The listing builds one solid part. Answer for the finished solid, in the listing's coordinates (mm). A direction names the side the tool comes from. Round coordinates to 2 decimals unless told otherwise and drop trailing zeros. Order: outer loops, then holes, each group sorted by start corner. A loop starts at its lowest first (then second) coordinate and runs counter-clockwise, first axis right, second up. Notation, with made-up numbers: (-2, 40.5) -> (55, 40.5) arc R25 ccw to (55, 78.5) -> close; hole circle Ø5 at (55.5, -21.5). An arc over 180 degrees is marked (long way). Answer in a Markdown table with one row per item. Add a question column.
Autodesk Inventor part; units mm, degrees
ref_plane "Work Plane1" through (0, 0, 0) normal (0, 0, 1) x (1, 0, 0)
ref_plane "YZ Plane" through (0, 0, 0) normal (1, 0, 0) x (0, 1, 0)
ref_plane "XZ Plane" through (0, 0, 0) normal (0, 1, 0) x (-1, 0, 0)
sketch "Sketch1" plane through (0, 0, 0) normal (0, 1, 0) x (-1, 0, 0)
  circle A0 centre (0, 0) radius 19
  arc A1 (16.9227, -16.3055) -> (-8.0375, -22.0828) centre (0, 0) ccw
  line L0 (0, 23.5) -> (0, -23.5) construction
  line L1 (23.5, 0) -> (-23.5, 0) construction
  line L2 (-8.0375, -22.0828) -> (11.2262, -29.0942)
  line L3 (11.2262, -29.0942) -> (16.9227, -16.3055)
  line L4 (0, 0) -> (-8.9052, -24.4669) construction
  line L5 (21.7083, 9) -> (27.7083, 9)
  line L6 (27.7083, 9) -> (27.7083, -9)
  line L7 (27.7083, -9) -> (21.7083, -9)
  line L8 (14, 18.8746) -> (14, 26)
  line L9 (14, 26) -> (-14, 26)
  line L10 (-14, 26) -> (-14, 18.8746)
  line L11 (-21.7083, 9) -> (-27.7083, 9)
  line L12 (-27.7083, 9) -> (-27.7083, -9)
  line L13 (-27.7083, -9) -> (-21.7083, -9)
  point P0 (-14, 22.4373)
  dimension "d1" = 47
  dimension "d0" = 20.5
  dimension "d2" = 38
  dimension "d5" = 20
  dimension "d7" = 14
  dimension "d8" = 18
  dimension "d9" = 6
  dimension "d10" = 28
  dimension "d11" = 18
  dimension "d32" = 6
  dimension "d33" = 17
extrude "Extrusion1" add sketch "Sketch1" along normal blind 10
sketch "Sketch2" plane through (-16.9227, 0, -16.3055) normal (-0.9135, 0, -0.4069) x (-0.4069, 0, 0.9135)
  line L0 (-14, 0) -> (-14, 10)
  point P0 (8.0089, 0)
  point P1 (-8, 3.373)
  dimension "d24" = 6
hole "Hole1" at (-13.6676, 3.373, -23.6133) direction (0.9135, 0, 0.4069) diameter 3 depth 9.5 counterbore diameter 5 counterbore depth 5
sketch "Sketch3" plane through (-21.7083, 0, -9) normal (0, 0, -1) x (-1, 0, 0)
  line L0 (6, 0) -> (6, 10)
  line L1 (0, 0) -> (6, 0)
  point P0 (-21.7083, 0)
  point P1 (3, 5)
  point P2 (6, 5)
  point P3 (3, 0)
hole "Hole2" at (-24.7083, 5, -9) direction (0, 0, 1) diameter 5 end through all
sketch "Sketch4" plane through (27.7083, 0, -9) normal (0, 0, -1) x (-1, 0, 0)
  line L0 (0, 0) -> (0, 10)
  line L1 (0, 0) -> (6, 0)
  point P0 (27.7083, 0)
  point P1 (3, 5)
  point P2 (0, 5)
  point P3 (3, 0)
hole "Hole3" at (24.7083, 5, -9) direction (0, 0, 1) diameter 5 end through all
sketch "Sketch5" plane through (-14, 0, 26) normal (0, 0, 1) x (1, 0, 0)
  line L0 (0, 0) -> (0, 10)
  line L1 (28, 0) -> (28, 10)
  point P0 (14, 0)
  point P1 (4, 5)
  point P2 (24, 5)
  point P3 (0, 5)
  point P4 (28, 5)
  dimension "d48" = 4
  dimension "d49" = 4
hole "Hole4" at (-10, 5, 26) at (10, 5, 26) direction (0, 0, -1) diameter 3.242 depth 6
ref_plane "Work Plane1" through (0, 0, 0) normal (0, 0, 1) x (1, 0, 0)
split_face "Split1"
properties part number "2051"
Item 1: Find the intervals of material crossed by probe 1 along X at (y, z) = (5, 23.95); probe 2 along X at (y, z) = (5, 1.5); probe 3 along X at (y, z) = (5, 3.75), in increasing order. Write a range as [from, to].
Item 2: The part is cut by section D-D, the plane z = 13.5. Give the vertices of the cut face in (x, y), and give its area (3 significant figures).
Item 3: A tool of negligible diameter and unlimited length cuts with its end or side. For faces 3 (the face through (-9.764, 3.894, -20.088)), 4 (the face through (-11.1, 6.19, 22.96)), 5 (the face through (26.1, 2.7, -9)), from which of +Z, -Z, +X, -X, +Y, -Y can it reach the whole face along a straight path? Write none if from no direction.
Item 4: Flat-ended cylindrical pins translate along their axes: P1, Ø5, axis at y = 9, z = -21, coming from the +X side; P2, Ø3, axis at x = -23.5, y = 5.5, coming from the +Z side; P3, Ø1, axis at x = 10, y = 6, coming from the +Z side. Find the tip coordinate at first contact, or state that the pin passes through.
Item 5: The part is cut by section C-C, the plane z = 22. Give the vertices of the cut face in (x, y).
Item 6: The part is cut by section A-A, the plane z = 0. Give the vertices of the cut face in (x, y), and give its area (3 significant figures).
Item 7: The part is cut by section B-B, the plane x = 0. Give the vertices of the cut face in (y, z).
Item 8: For a pull along Y with two mould halves and no side action, classify faces 1 (the face through (23.3, 2.7, 9)), 2 (the face through (-4.998, 3.352, -19.729)) as released by +Y, released by -Y, zero draft, split by the parting line, or undercut.
Resolved:
| question | item | result |
|---|---|---|
| 1 | probe 1 | [-14, -11.62], [-8.38, 8.38], [11.62, 14] |
| 1 | probe 2 | [-27.71, -27.21], [-22.21, -18.94], [18.94, 22.21], [27.21, 27.71] |
| 1 | probe 3 | [-27.71, -27.21], [-22.21, -18.63], [18.63, 22.21], [27.21, 27.71] |
| 2 | outline | (-19.24, 0) -> (-13.37, 0) -> (-13.37, 10) -> (-19.24, 10) -> close; (13.37, 0) -> (19.24, 0) -> (19.24, 10) -> (13.37, 10) -> close |
| 2 | area | 117 mm2 |
| 3 | face 3 | none |
| 3 | face 4 | +Z |
| 3 | face 5 | -Z, +X, +Y, -Y |
| 4 | P1 | x = 14.49 |
| 4 | P2 | z = 9 |
| 4 | P3 | z = 20 |
| 5 | outline | (-14, 0) -> (14, 0) -> (14, 10) -> (-14, 10) -> close; hole circle Ø3.24 at (-10, 5); hole circle Ø3.24 at (10, 5) |
| 6 | outline | (-27.71, 0) -> (-19, 0) -> (-19, 10) -> (-27.71, 10) -> close; (19, 0) -> (27.71, 0) -> (27.71, 10) -> (19, 10) -> close; hole circle Ø5 at (-24.71, 5); hole circle Ø5 at (24.71, 5) |
| 6 | area | 135 mm2 |
| 7 | outline | (0, -25.01) -> (10, -25.01) -> (10, -19) -> (0, -19) -> close; (0, 19) -> (10, 19) -> (10, 26) -> (0, 26) -> close |
| 8 | face 1 | zero draft |
| 8 | face 2 | undercut |
